Here's how the part is built. I have some questions about the finished solid (model axes, mm). Face numbers are marked on the shaded views. A direction names the side the tool comes from. Round coordinates to 2 decimals unless told otherwise and drop trailing zeros. Order: outer loops, then holes, each group sorted by start corner. A loop starts at its lowest first (then second) coordinate and runs counter-clockwise, first axis right, second up. Notation, with made-up numbers: M -39.5,86 L 10.5,86 A25 cw 10.5,100 Z; hole C 47.5,14.5 d1. An arc over 180 degrees is marked long. Write item = value, one per line. Start each with the question number.
Item 1: I want a section at A-A, the plane y = 11.5. List the corners of the cut face in (x, z) for me, plus the area to 3 significant figures.
Item 2: I want a section at B-B, the plane y = 9.5. List the corners of the cut face in (x, z) for me.
Item 3: Please list where these lines run through material, in increasing order: L1, parallel to X at y = 8, z = -6.25; L2, parallel to Z at x = 1, y = 4.75; L3, parallel to Z at x = 1.75, y = 5.25.
Item 4: I'm going to push flat-ended pins straight in: P1, Ø1, axis at y = 8, z = -2.5, coming from the -X side; P2, Ø8, axis at x = 3.5, y = 6.5, coming from the -Z side; P3, Ø8, axis at y = 8.5, z = 4, coming from the -X side. Where does each tip first touch, or does it pass through?
Item 5: For the marked faces 1 and 2, which set-ups out of +Z, -Z, +X, -X, +Y, -Y let a thin tool reach every point of the face, with its end or its side?
```python
from build123d import *

# Parameters (mm, degrees)
IZIM2_R               = 1.25
KES_EKSTR_ZYON1_DEPTH = 10


with BuildPart() as part:
    # Çizim1 → Döndür3 (revolve)
    with BuildSketch(Plane(origin=(0, 0, 0), x_dir=(0, 0, -1), z_dir=(1, 0, 0)), mode=Mode.PRIVATE) as d_nd_r3_sk:
        with BuildLine():
            Line((0, 1.4985), (0, 0))
            Line((0, 0), (1.24875, 0))
            Line((1.24875, 0), (4.868655858, 0))
            ThreePointArc((4.868655858, 0), (5.951824945, 0.454850463), (6.993, 0.999))
            Line((6.993, 0.999), (11.838744981, 0.999))
            Line((11.838744981, 0.999), (12.913678251, 0.999))
            Line((12.913678251, 0.999), (12.896228404, 1.284302481))
            Line((12.896228404, 1.284302481), (12.058257846, 14.985))
            Line((12.058257846, 14.985), (9.876973107, 14.985))
            ThreePointArc((9.876973107, 14.985), (8.649440213, 8.487771762), (3.632727273, 4.180405623))
            ThreePointArc((3.632727273, 4.180405623), (3.171102899, 3.813308184), (2.997, 3.249796185))
            Line((2.997, 3.249796185), (2.997, 1.4985))
            Line((2.997, 1.4985), (1.24875, 1.4985))
            Line((1.24875, 1.4985), (0, 1.4985))
        make_face()
    revolve(d_nd_r3_sk.sketch.rotate(Axis((0, 1.4985, 0), (0, -1, 0)), 180), axis=Axis((0, 1.4985, 0), (0, -1, 0)))

    # Çizim2 → Kes-Ekstrüzyon1 (cut)
    with BuildSketch(Plane.XZ):
        with Locations(Location((0, 0, 0), (0, 0, 270))):
            Circle(IZIM2_R)
    extrude(amount=-KES_EKSTR_ZYON1_DEPTH, mode=Mode.SUBTRACT)


solid = part.part
```
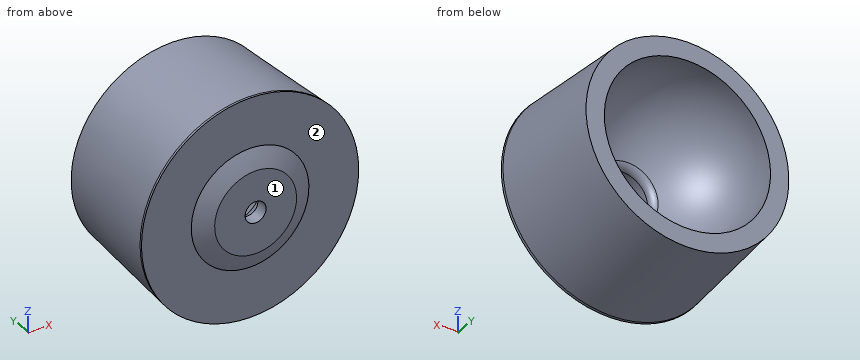
Filled in:
q1.outline = C 0,0 d24.54; hole C 0,0 d19.58
q1.area = 172 mm^2
q2.outline = C 0,0 d24.79; hole C 0,0 d18.32
q3.L1 = -10.81 to -5.53, 5.53 to 10.81
q3.L2 = -12.64 to -4.74, 4.74 to 12.64
q3.L3 = -12.53 to -5.38, 5.38 to 12.53
q4.P1 = -12.33
q4.P2 = -12.73
q4.P3 = -12.58
q5.face_1 = +Z, -Z, +X, -X, -Y
q5.face_2 = -Y
